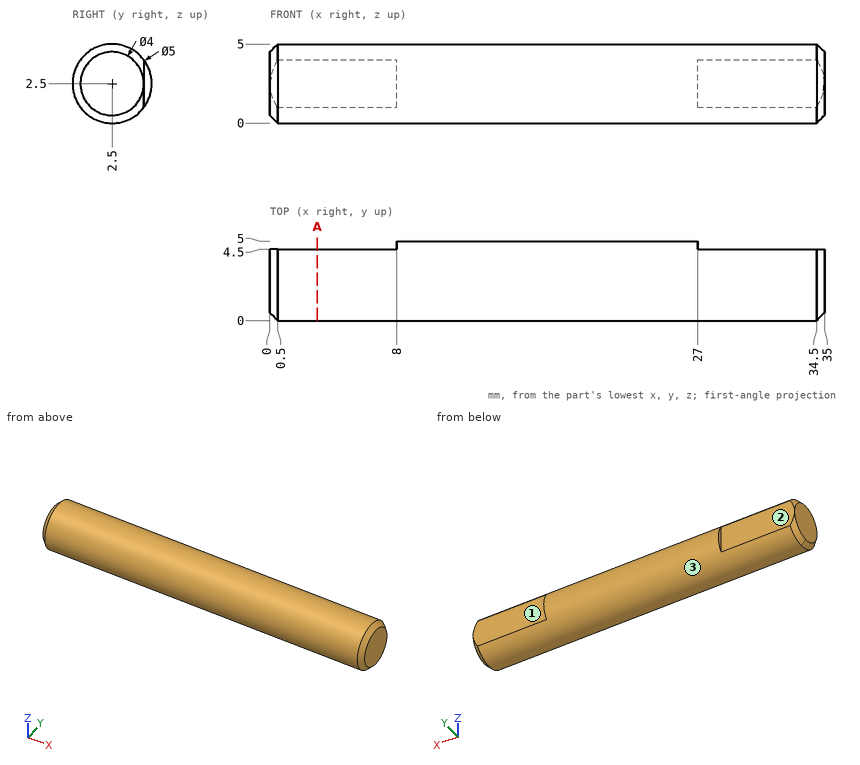
The figure shows three views and two pictorial views of one solid part (mm, origin at its lowest corner). Answer the questions. A direction names the side the tool comes from. Give positions to 0.01 mm unless a question says otherwise; leave off trailing zeros. Order: outer loops, then holes, each group sorted by start corner. A loop starts at its lowest first (then second) coordinate and runs counter-clockwise, first axis right, second up. Notation, with made-up numbers: (47, 49.5) -> (104, 49.5) arc R22 ccw to (104, 81.5) -> close; hole circle Ø7 at (34, -1). An arc over 180 degrees is marked (long way). One line per item, written item: value.
1) Find section A-A, the plane x = 3. Determine the outline of the cut face in (y, z), plus the area to 3 significant figures.
Reported:
outline: (4.5, 1) -> (4.5, 4) arc R2.5 ccw (long way) to start
area: 18.6 mm^2
2) A tool of negligible diameter and unlimited length cuts with its end or side. For the marked faces 1, 2 and 3, from which of +Z, -Z, +X, -X, +Y, -Y can it reach the whole face along a straight path? Write none if from no direction.
Reported:
face 1: +Z, -Z, +X, +Y
face 2: +Z, -Z, -X, +Y
face 3: +X, -X
3) Find the intervals of material crossed by line 1 (Z direction, x = 13.5, y = 2.65); line 2 (Y direction, x = 6, z = 4); line 3 (Y direction, x = 21.5, z = 2.75), in increasing order.
Reported:
line 1: z = 0 to 5
line 2: y = 0.5 to 4.5
line 3: y = 0.01 to 4.99
